Autodesk Inventor part; units mm, degrees
ref_plane "YZ Plane" through (0, 0, 0) normal (1, 0, 0) x (0, 1, 0)
ref_plane "XZ Plane" through (0, 0, 0) normal (0, 1, 0) x (-1, 0, 0)
ref_plane "XY Plane" through (0, 0, 0) normal (0, 0, 1) x (1, 0, 0)
sketch "Sketch1" plane through (0, 0, 0) normal (0, 0, 1) x (1, 0, 0)
  circle A0 centre (0, 0) radius 2.5
  line L0 (-7.3323, 0) -> (-3.6662, 6.35)
  line L1 (-3.6662, 6.35) -> (3.6662, 6.35)
  line L2 (3.6662, 6.35) -> (7.3323, 0)
  line L3 (7.3323, 0) -> (3.6662, -6.35)
  line L4 (3.6662, -6.35) -> (-3.6662, -6.35)
  line L5 (-3.6662, -6.35) -> (-7.3323, 0)
  dimension "d0" = 5
  dimension "d1" = 12.7
extrude "Extrusion1" add sketch "Sketch1" along normal blind 79.835
chamfer "Chamfer1" distance 0.5 angle 45 12 edges at (0, -6.35, 0) (-5.4993, -3.175, 0) (-5.4993, 3.175, 0) (0, 6.35, 0) (5.4993, 3.175, 0) (5.4993, -3.175, 0) (0, -6.35, 79.835) (5.4993, -3.175, 79.835) (5.4993, 3.175, 79.835) (0, 6.35, 79.835) (-5.4993, 3.175, 79.835) (-5.4993, -3.175, 79.835)
properties part number "spacers"
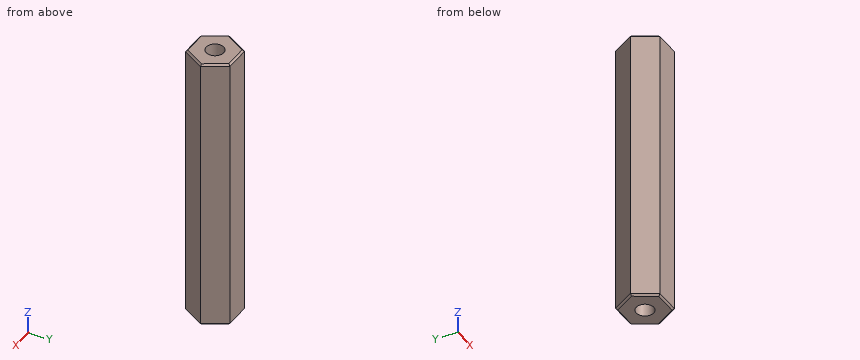
Read the model definition and answer for the solid it produces. Units are mm, in the model's axes. Coordinates: 2 decimals unless noted, no trailing zeros. Write each loop counter-clockwise with the first axis right and the second up, starting at its lowest first coordinate (ties: lowest second). Pieces come first, ordered by that corner, then holes. Notation, with made-up numbers: (81, 69.5) -> (115, 69.5) arc R31 ccw to (115, 102.5) -> close; hole circle Ø10 at (-15.75, -32.5). An arc over 180 degrees is marked (long way). Answer as a JSON object with one key per item and string values.
Q1. The part is cut by section A-A on x = 0. Give the vertices of the cut face in (y, z) (3 decimals).
The answers:
{"outline": "(-6.35, 0.5) -> (-5.85, 0) -> (-2.5, 0) -> (-2.5, 79.835) -> (-5.85, 79.835) -> (-6.35, 79.335) -> close; (2.5, 0) -> (5.85, 0) -> (6.35, 0.5) -> (6.35, 79.335) -> (5.85, 79.835) -> (2.5, 79.835) -> close"}
Q2. Flat-ended cylindrical pins translate along their axes: pin 1 Ø6 at (x, y) = (0, 0) entering from -Z; pin 2 Ø1 at (y, z) = (-2, 65.5) entering from +X. Find the tip coordinate at first contact, or state that the pin passes through.
The answers:
{"pin 1": "stops at z = 0", "pin 2": "stops at x = 6.47"}
Q3. Consider line 1 (Y direction, x = 0, z = 46); line 2 (Y direction, x = -2, z = 38); line 3 (X direction, y = 2.25, z = 44.5). Determine where each line is inside the solid, lowest interval first. Write a range as [from, to].
The answers:
{"line 1": "y = [-6.35, -2.5], [2.5, 6.35]", "line 2": "y = [-6.35, -1.5], [1.5, 6.35]", "line 3": "x = [-6.03, -1.09], [1.09, 6.03]"}
Q4. The part is cut by section D-D on x = 4.5. Give the vertices of the cut face in (y, z) (3 decimals).
The answers:
{"outline": "(-4.906, 0.5) -> (-3.906, 0) -> (3.906, 0) -> (4.906, 0.5) -> (4.906, 79.335) -> (3.906, 79.835) -> (-3.906, 79.835) -> (-4.906, 79.335) -> close"}
Q5. The part is cut by section B-B on z = 23. Give the vertices of the cut face in (x, y).
The answers:
{"outline": "(-7.33, 0) -> (-3.67, -6.35) -> (3.67, -6.35) -> (7.33, 0) -> (3.67, 6.35) -> (-3.67, 6.35) -> close; hole circle Ø5 at (0, 0)"}
Q6. The part is cut by section C-C on y = -5. Give the vertices of the cut face in (x, z) (3 decimals).
The answers:
{"outline": "(-4.446, 0.5) -> (-3.868, 0) -> (3.868, 0) -> (4.446, 0.5) -> (4.446, 79.335) -> (3.868, 79.835) -> (-3.868, 79.835) -> (-4.446, 79.335) -> close"}
